Source: CAD feature listing. Evaluate the final solid. Frame: model axes, mm. A direction names the side the tool comes from. Give positions to 0.01 mm unless a question says otherwise; leave off trailing zeros. Write each loop counter-clockwise with the first axis right and the second up, starting at its lowest first coordinate (ties: lowest second). Pieces come first, ordered by that corner, then holes.
```python
from build123d import *

# Parameters (mm, degrees)
F0_W     = 260
F0_H     = 260
F1_DEPTH = 1
F0_H_2   = 20
F0_W_2   = 20
F2_DEPTH = 5
F3_DEPTH = 5


with BuildPart() as f1:
    # F0 (on Front) → F1 (new body)
    with BuildSketch(Plane.XZ):
        with Locations((-71.63621746, -55.5927120769)):
            Rectangle(F0_W, F0_H)
    extrude(amount=F1_DEPTH)

    # F0 (on Front) → F2 (join)
    with BuildSketch(Plane.XZ):
        with Locations((-71.63621746, 84.4072879231)):
            Rectangle(F0_W, F0_H_2)
        with Locations((68.36378254, 84.4072879231)):
            Rectangle(F0_W_2, F0_H_2)
        with Locations((68.36378254, -55.5927120769)):
            Rectangle(F0_W_2, F0_H)
        with Locations((68.36378254, -195.5927120769)):
            Rectangle(F0_W_2, F0_H_2)
        with Locations((-71.63621746, -195.5927120769)):
            Rectangle(F0_W, F0_H_2)
        with Locations((-211.63621746, -195.5927120769)):
            Rectangle(F0_W_2, F0_H_2)
        with Locations((-211.63621746, -55.5927120769)):
            Rectangle(F0_W_2, F0_H)
        with Locations((-211.63621746, 84.4072879231)):
            Rectangle(F0_W_2, F0_H_2)
    extrude(amount=F2_DEPTH)

    # F0 (on Front) → F3 (join)
    with BuildSketch(Plane.XZ):
        with Locations((-71.63621746, 84.4072879231)):
            Rectangle(F0_W, F0_H_2)
        with Locations((68.36378254, 84.4072879231)):
            Rectangle(F0_W_2, F0_H_2)
        with Locations((68.36378254, -55.5927120769)):
            Rectangle(F0_W_2, F0_H)
        with Locations((68.36378254, -195.5927120769)):
            Rectangle(F0_W_2, F0_H_2)
        with Locations((-71.63621746, -195.5927120769)):
            Rectangle(F0_W, F0_H_2)
        with Locations((-211.63621746, -195.5927120769)):
            Rectangle(F0_W_2, F0_H_2)
        with Locations((-211.63621746, -55.5927120769)):
            Rectangle(F0_W_2, F0_H)
        with Locations((-211.63621746, 84.4072879231)):
            Rectangle(F0_W_2, F0_H_2)
    extrude(amount=-F3_DEPTH)


solid = f1.part
```
1. Cut plane A-A, the plane y = 1.5. Return the cut outline in (x, z).
2. Mould query, pull axis Z, two halves, no side actions, for faces 1 (the flat face through (-74, 0, -205.593)), 2 (the flat face through (-73, 0, -54)), 3 (the flat face through (-74, -5, -187)). Classes: +Z half, -Z half, draft (parallel to the pull), parting line (faces both ways), or undercut.
3. Cut plane C-C, the plane x = -173. Return the cut outline in (y, z).
4. Line query: L1, parallel to X at y = 3.75, z = -20; L2, parallel to Z at x = -71, y = 0.5; L3, parallel to Y at x = -64.5, z = 45. Output: solid intervals per line, ascending.
5. Contact query for a flat-ended pin moving along its axis: P1, Ø3, axis at x = -65, z = -43, coming from the +Y side. Output: stop coordinate, or through.
6. Cut plane B-B, the plane z = -24.5. Return the cut outline in (x, y), then the cut area to 3 significant figures.
7. Access query for faces 4 (the flat face through (-74, 5, -187)), 5 (the flat face through (-73, -1, -54)). Directions: +Z, -Z, +X, -X, +Y, -Y. A direction counts if a zero-diameter tool reaches every point of the face in a straight line with its end or side. Return the directions, or none.
Response values:
1. outline: (-221.64, -205.59) - (78.36, -205.59) - (78.36, 94.41) - (-221.64, 94.41) - close; hole (-201.64, -185.59) - (58.36, -185.59) - (58.36, 74.41) - (-201.64, 74.41) - close
2. face 1: -Z half
2. face 2: undercut
2. face 3: draft
3. outline: (-5, -205.59) - (5, -205.59) - (5, -185.59) - (0, -185.59) - (0, 74.41) - (5, 74.41) - (5, 94.41) - (-5, 94.41) - (-5, 74.41) - (-1, 74.41) - (-1, -185.59) - (-5, -185.59) - close
4. L1: x = -221.64 to -201.64, 58.36 to 78.36
4. L2: z = -205.59 to -185.59, 74.41 to 94.41
4. L3: y = -1 to 0
5. P1: stops at y = 0
6. outline: (-221.64, -5) - (-201.64, -5) - (-201.64, -1) - (58.36, -1) - (58.36, -5) - (78.36, -5) - (78.36, 5) - (58.36, 5) - (58.36, 0) - (-201.64, 0) - (-201.64, 5) - (-221.64, 5) - close
6. area: 660 mm2
7. face 4: +Z, -Z, +X, -X, +Y
7. face 5: -Y
